Here's how the part is built. I have some questions about the finished solid (model axes, mm). Face numbers are marked on the shaded views. A direction names the side the tool comes from. Round coordinates to 2 decimals unless told otherwise and drop trailing zeros. Write each loop counter-clockwise with the first axis right and the second up, starting at its lowest first coordinate (ties: lowest second). Pieces come first, ordered by that corner, then holes. Notation, with made-up numbers: (76.5, -11.75) - (126.5, -11.75) arc R11 ccw to (126.5, 2.25) - close; hole circle Ø2 at (60.25, 51). An arc over 180 degrees is marked (long way). Return JSON: item names as keys, results as strings. Group by question number.
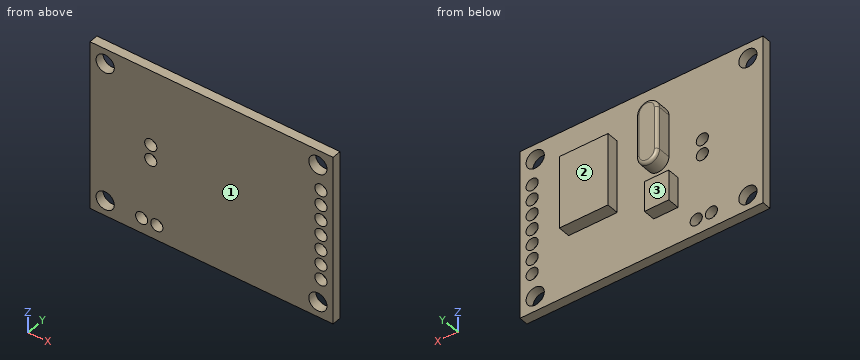
```python
from build123d import *

# Parameters (mm, degrees)
SKETCH1_W           = 40
SKETCH1_H           = 28
SKETCH1_R           = 1.5
BOSS_EXTRUDE1_DEPTH = 1.5
SKETCH2_R           = 1
CUT_EXTRUDE1_DEPTH  = 2.5
SKETCH3_W           = 8
SKETCH3_H           = 12
BOSS_EXTRUDE2_DEPTH = 2
SKETCH4_W           = 4
SKETCH4_H           = 5
BOSS_EXTRUDE3_DEPTH = 2
SKETCH5_R           = 1
CUT_EXTRUDE2_DEPTH  = 2.5
BOSS_EXTRUDE4_DEPTH = 2.5
FILLET1_R           = 0.5


with BuildPart() as part:
    # Sketch1 → Boss-Extrude1 (new body)
    with BuildSketch(Plane(origin=(0, 0, 0), x_dir=(1, 0, 0), z_dir=(0, 1, 0))):
        with Locations((20, 14)):
            Rectangle(SKETCH1_W, SKETCH1_H)
        with Locations((2.5, 25.5)):
            Circle(SKETCH1_R, mode=Mode.SUBTRACT)
        with Locations((2.5, 2.5)):
            Circle(SKETCH1_R, mode=Mode.SUBTRACT)
        with Locations((37.5, 25.5)):
            Circle(SKETCH1_R, mode=Mode.SUBTRACT)
        with Locations((37.5, 2.5)):
            Circle(SKETCH1_R, mode=Mode.SUBTRACT)
    extrude(amount=BOSS_EXTRUDE1_DEPTH)

    # Sketch2 → Cut-Extrude1 (cut, through all)
    with BuildSketch(Plane(origin=(0, 1.5, 0), x_dir=(1, 0, 0), z_dir=(0, 1, 0))):
        with Locations((38, 6.5)):
            Circle(SKETCH2_R)
        with Locations((38, 9)):
            Circle(SKETCH2_R)
        with Locations((38, 11.5)):
            Circle(SKETCH2_R)
        with Locations((38, 14)):
            Circle(SKETCH2_R)
        with Locations((38, 16.5)):
            Circle(SKETCH2_R)
        with Locations((38, 19)):
            Circle(SKETCH2_R)
        with Locations((38, 21.5)):
            Circle(SKETCH2_R)
    extrude(amount=-CUT_EXTRUDE1_DEPTH, mode=Mode.SUBTRACT)

    # Sketch3 → Boss-Extrude2 (add)
    with BuildSketch(Plane(origin=(0, 1.5, 0), x_dir=(1, 0, 0), z_dir=(0, 1, 0))):
        with Locations((28, 12)):
            Rectangle(SKETCH3_W, SKETCH3_H)
    extrude(amount=BOSS_EXTRUDE2_DEPTH)

    # Sketch4 → Boss-Extrude3 (add)
    with BuildSketch(Plane(origin=(0, 1.5, 0), x_dir=(1, 0, 0), z_dir=(0, 1, 0))):
        with Locations((16, 19.5)):
            Rectangle(SKETCH4_W, SKETCH4_H)
    extrude(amount=BOSS_EXTRUDE3_DEPTH)

    # Sketch5 → Cut-Extrude2 (cut, through all)
    with BuildSketch(Plane(origin=(0, 1.5, 0), x_dir=(1, 0, 0), z_dir=(0, 1, 0))):
        with Locations((10, 15)):
            Circle(SKETCH5_R)
        with Locations((10, 12.5)):
            Circle(SKETCH5_R)
        with Locations((8.5, 25.5)):
            Circle(SKETCH5_R)
        with Locations((11, 25.5)):
            Circle(SKETCH5_R)
    extrude(amount=-CUT_EXTRUDE2_DEPTH, mode=Mode.SUBTRACT)

    # Sketch6 → Boss-Extrude4 (add)
    with BuildSketch(Plane(origin=(0, 1.5, 0), x_dir=(1, 0, 0), z_dir=(0, 1, 0))):
        with BuildLine():
            Line((19, 12.75), (19, 5.75))
            ThreePointArc((19, 5.75), (17.25, 4), (15.5, 5.75))
            Line((15.5, 5.75), (15.5, 12.75))
            ThreePointArc((15.5, 12.75), (17.25, 14.5), (19, 12.75))
        make_face()
    extrude(amount=BOSS_EXTRUDE4_DEPTH)

    # Fillet1
    fillet1_edges = [part.edges().sort_by_distance(p)[0] for p in [
        (17.25, 4, -14.5),
        (15.5, 4, -9.25),
        (17.25, 4, -4),
        (19, 4, -9.25),
    ]]
    fillet(fillet1_edges, radius=FILLET1_R)


solid = part.part
```
1) I need wall thicknesses on line 1 along X through (y, z) = (0.65, -25.5); line 2 along X through (y, z) = (0.4, -19); line 3 along Z through (x, y) = (8.5, 1). Which ranges of each line are inside material? Lowest first, please.
2) Imagine slicing it at C-C (x = 2.5). Please give me the cut outline in (y, z).
3) Imagine slicing it at A-A (z = -21.5). Please give me the cut outline in (x, y).
4) Imagine slicing it at B-B (y = 0.95). Give the number of separate pieces and of enclosed holes in the cut face, plus the area to 3 significant figures.
5) Will these pins go through, and if not, where does the flat tip stop? pin 1 Ø1.2 at (x, z) = (38, -19) entering from +Y; pin 2 Ø1 at (x, y) = (17, 2.5) entering from -Z; pin 3 Ø1 at (y, z) = (2.5, -12.5) entering from -X; pin 4 Ø1.6 at (y, z) = (3, -20.5) entering from -X.
6) For the marked faces 1, 2 and 3, which set-ups out of +Z, -Z, +X, -X, +Y, -Y let a thin tool reach every point of the face, with its end or its side?
7) Imagine slicing it at D-D (z = -26). Please give me the cut outline in (x, y), plus the area to 3 significant figures.
Results found:
{
 "1": {"line 1": "x = 0 to 1, 4 to 7.5, 9.5 to 10, 12 to 36, 39 to 40", "line 2": "x = 0 to 37, 39 to 40", "line 3": "z = -28 to -26.5, -24.5 to 0"},
 "2": {"outline": "(0, -28) - (1.5, -28) - (1.5, -27) - (0, -27) - close; (0, -24) - (1.5, -24) - (1.5, -4) - (0, -4) - close; (0, -1) - (1.5, -1) - (1.5, 0) - (0, 0) - close"},
 "3": {"outline": "(0, 0) - (37, 0) - (37, 1.5) - (18, 1.5) - (18, 3.5) - (14, 3.5) - (14, 1.5) - (0, 1.5) - close; (39, 0) - (40, 0) - (40, 1.5) - (39, 1.5) - close"},
 "4": {"separate pieces": "1", "enclosed holes": "15", "area": "1,060 mm²"},
 "5": {"pin 1": "passes through", "pin 2": "stops at z = -22", "pin 3": "stops at x = 15.5", "pin 4": "stops at x = 14"},
 "6": {"face 1": "+Z, -Z, +X, -X, -Y", "face 2": "+Z, -Z, +X, +Y", "face 3": "-Z, +X, -X, +Y"},
 "7": {"outline": "(0, 0) - (1.09, 0) - (1.09, 1.5) - (0, 1.5) - close; (3.91, 0) - (7.63, 0) - (7.63, 1.5) - (3.91, 1.5) - close; (9.37, 0) - (10.13, 0) - (10.13, 1.5) - (9.37, 1.5) - close; (11.87, 0) - (36.09, 0) - (36.09, 1.5) - (11.87, 1.5) - close; (38.91, 0) - (40, 0) - (40, 1.5) - (38.91, 1.5) - close", "area": "46.3 mm²"}
}
